The model under review builds one solid part; all positions refer to its coordinate system, in mm. Face numbers are marked on the shaded views. A direction names the side the tool comes from. Give positions to 0.01 mm unless a question says otherwise; leave off trailing zeros. Order: outer loops, then holes, each group sorted by start corner. A loop starts at its lowest first (then second) coordinate and runs counter-clockwise, first axis right, second up. Notation, with made-up numbers: (6, 83.5) - (18, 83.5) arc R18 ccw to (18, 87.5) - close; hole circle Ø7 at (36, 43.5). An arc over 180 degrees is marked (long way). Put each result on its own line as item: value.
```python
from build123d import *

# Parameters (mm, degrees)
BOSS_EXTRUDE1_DEPTH = 10
SKETCH2_R           = 1.997822351
SKETCH2_R_2         = 2.000000328
CUT_EXTRUDE1_DEPTH  = 107.961093012


with BuildPart() as part:
    # Sketch1 → Boss-Extrude1 (new body)
    with BuildSketch(Plane(origin=(0, 0, 0), x_dir=(1, 0, 0), z_dir=(0, 1, 0))):
        Polygon((-32.812912017, 69.703683257), (-20.812911913, 69.703683257), (-20.812911913, 72.703689337), (-8.812911808, 72.703689337), (-8.812911808, 69.703683257), (3.187088063, 69.703683257), (3.187088063, 72.703689337), (15.1870884, 72.703689337), (15.1870884, 69.703683257), (27.187088504, 69.703683257), (27.187088504, 72.703689337), (39.187088609, 72.703689337), (39.187088609, 69.703683257), (51.18708685, 69.703683257), (51.18708685, 72.703689337), (69.187089801, 72.703689337), (69.187089801, 69.703683257), (69.187089801, 64.03671205), (72.18708843, 64.03671205), (72.18708843, 53.703688085), (69.187089801, 53.703688085), (69.187089801, 40.036708117), (72.18708843, 40.036708117), (72.18708843, 29.703684151), (69.187089801, 29.703684151), (69.187089801, 22.703684866), (-74.812911451, 22.703684866), (-74.812911451, 29.703684151), (-77.81291008, 29.703684151), (-77.81291008, 40.036708117), (-74.812911451, 40.036708117), (-74.812911451, 53.703688085), (-77.81291008, 53.703688085), (-77.81291008, 64.03671205), (-74.812911451, 64.03671205), (-74.812911451, 69.703683257), (-74.812911451, 72.703689337), (-56.812912226, 72.703689337), (-56.812912226, 69.703683257), (-44.812910259, 69.703683257), (-44.812910259, 72.703689337), (-32.812912017, 72.703689337), align=None)
    extrude(amount=BOSS_EXTRUDE1_DEPTH)

    # Sketch2 → Cut-Extrude1 (cut, through all)
    with BuildSketch(Plane(origin=(0, 10, 0), x_dir=(1, 0, 0), z_dir=(0, 1, 0))):
        with Locations(Location((-19.704415408, 45.837319398, 0), (0, 0, 270))):
            Circle(SKETCH2_R)
        with Locations(Location((19.706618041, 45.84139958, 0), (0, 0, 270))):
            Circle(SKETCH2_R_2)
    extrude(amount=-CUT_EXTRUDE1_DEPTH, mode=Mode.SUBTRACT)


solid = part.part
```
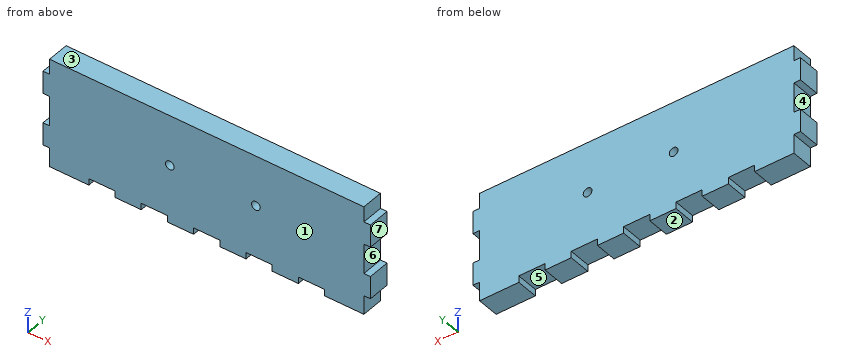
(1) The part is to be moulded in two halves that separate along Z. For the marked faces 1, 2, 3 and 4, say which applies: pulls with the +Z half, pulls with the -Z half, needs draft (parallel to the pull), parting line crosses it, or undercut.
The answers:
face 1: needs draft
face 2: pulls with the -Z half
face 3: pulls with the +Z half
face 4: undercut
(2) Wall thickness on L1, parallel to Z at x = 19.5, y = 7; L2, parallel to X at y = 1.25, z = -45; L3, parallel to Z at x = 0.5, y = 4.25: over which ranges is each line inside the solid? List them lowest first.
The answers:
L1: -69.7 to -47.83, -43.85 to -22.7
L2: -74.81 to -21.52, -17.89 to 17.89, 21.52 to 69.19
L3: -69.7 to -22.7
(3) Take a section at A-A, the plane z = -46. Write out the cut boundary in (x, y).
The answers:
outline: (-74.81, 0) - (-21.7, 0) - (-21.7, 10) - (-74.81, 10) - close; (-17.71, 0) - (17.71, 0) - (17.71, 10) - (-17.71, 10) - close; (21.7, 0) - (69.19, 0) - (69.19, 10) - (21.7, 10) - close
(4) Clearance check with flat-ended pins moving along their axes: pin 1 Ø1.5 at (y, z) = (4, -71.5) entering from -X; pin 2 Ø3.5 at (x, y) = (-77, 5.5) entering from +Z; pin 3 Ø5 at (x, y) = (-4.5, 6) entering from -Z; pin 4 Ø10 at (x, z) = (-18, -32.5) entering from -Y. State where each tip first meets the part, or that it passes through.
The answers:
pin 1: x = -74.81
pin 2: z = -29.7
pin 3: z = -69.7
pin 4: y = 0
(5) For the marked faces 5, 6 and 7, list the 3-axis set-ups (+Z, -Z, +X, -X, +Y, -Y) from which the entire face can be reached by the end or side of a thin tool; tool diameter is ignored.
The answers:
face 5: -Z, +Y, -Y
face 6: +X, +Y, -Y
face 7: +Z, -Z, +X, +Y, -Y
(6) Take a section at B-B, the plane y = 1.75. Count the separate pieces of the cut face and the enclosed holes in it, then the cut area to 3 significant figures.
The answers:
separate pieces: 1
enclosed holes: 2
area: 7,120 mm^2
